```python
from build123d import *

# Parameters (mm, degrees)
V3_BOX_FOOTPRINT_100_X_45_MM_W                 = 100
V3_BOX_FOOTPRINT_100_X_45_MM_H                 = 45
V3_BOX_HEIGHT_35_MM_DEPTH                      = 35
V3_REAR_OPENING_96_X_31_MM_W                   = 96
V3_REAR_OPENING_96_X_31_MM_H                   = 31
V3_CAVITY_ALL_WALLS_2_MM_DEPTH                 = 43
V3_SQUARE_BEAMS_10_X_10_PITCH_95_MM_W          = 10
V3_SQUARE_BEAMS_10_X_10_PITCH_95_MM_H          = 10
V3_FORWARD_BEAM_LENGTH_65_MM_DEPTH             = 65
V3_LEFT_PCB_EAR_PROFILE_W                      = 10
V3_LEFT_PCB_EAR_PROFILE_H                      = 10
V3_LEFT_INWARD_EAR_5_MM_DEPTH                  = 5
V3_RIGHT_PCB_EAR_PROFILE_W                     = 10
V3_RIGHT_PCB_EAR_PROFILE_H                     = 10
V3_RIGHT_INWARD_EAR_5_MM_DEPTH                 = 5
V3_PCB_ROOF_PAIR_PITCH_85_MM_R                 = 1.7
V3_M3_ROOF_HOLES_DIAMETER_3_4_MM_DEPTH         = 2
V3_PCB_FORWARD_PAIR_ROW_SPACING_60_MM_R        = 1.7
V3_M3_PCB_EAR_HOLES_DEPTH                      = 10
V3_CHASSIS_TOP_HOLES_WIDTH_95_DEPTH_40_M_R     = 1.7
V3_M3_BEAM_TOP_BOTTOM_HOLES_DEPTH              = 10
V3_HANGING_PLATE_OFFSET_26_THICKNESS_2_5_W     = 110
V3_HANGING_PLATE_OFFSET_26_THICKNESS_2_5_H     = 2.5
V3_MOUNTING_PLATE_DOWNWARD_15_MM_WIDTH_1_DEPTH = 15
V3_FOUR_MOUNTING_SLOTS_3_4_X_10_MM_DEPTH       = 2.5


with BuildPart() as part:
    # V3 box footprint 100 x 45 mm → V3 box height 35 mm (new body)
    with BuildSketch(Plane.XY):
        with Locations((0, 22.5)):
            Rectangle(V3_BOX_FOOTPRINT_100_X_45_MM_W, V3_BOX_FOOTPRINT_100_X_45_MM_H)
    extrude(amount=V3_BOX_HEIGHT_35_MM_DEPTH)

    # V3 rear opening 96 x 31 mm → V3 cavity all walls 2 mm (cut)
    with BuildSketch(Plane(origin=(0, 45, 0), x_dir=(1, 0, 0), z_dir=(0, 1, 0))):
        with Locations((0, -17.5)):
            Rectangle(V3_REAR_OPENING_96_X_31_MM_W, V3_REAR_OPENING_96_X_31_MM_H)
    extrude(amount=-V3_CAVITY_ALL_WALLS_2_MM_DEPTH, mode=Mode.SUBTRACT)

    # V3 square beams 10 x 10 pitch 95 mm → V3 forward beam length 65 mm (add)
    with BuildSketch(Plane.XZ):
        with Locations((-47.5, 30)):
            Rectangle(V3_SQUARE_BEAMS_10_X_10_PITCH_95_MM_W, V3_SQUARE_BEAMS_10_X_10_PITCH_95_MM_H)
        with Locations((47.5, 30)):
            Rectangle(V3_SQUARE_BEAMS_10_X_10_PITCH_95_MM_W, V3_SQUARE_BEAMS_10_X_10_PITCH_95_MM_H)
    extrude(amount=V3_FORWARD_BEAM_LENGTH_65_MM_DEPTH)

    # V3 left PCB ear profile → V3 left inward ear 5 mm (add)
    with BuildSketch(Plane(origin=(-42.5, 0, 0), x_dir=(0, 0, -1), z_dir=(1, 0, 0))):
        with Locations((-30, -20)):
            Rectangle(V3_LEFT_PCB_EAR_PROFILE_W, V3_LEFT_PCB_EAR_PROFILE_H)
    extrude(amount=V3_LEFT_INWARD_EAR_5_MM_DEPTH)

    # V3 right PCB ear profile → V3 right inward ear 5 mm (add)
    with BuildSketch(Plane.ZY.offset(-42.5)):
        with Locations((30, -20)):
            Rectangle(V3_RIGHT_PCB_EAR_PROFILE_W, V3_RIGHT_PCB_EAR_PROFILE_H)
    extrude(amount=V3_RIGHT_INWARD_EAR_5_MM_DEPTH)

    # V3 PCB roof pair pitch 85 mm → V3 M3 roof holes diameter 3.4 mm (cut)
    with BuildSketch(Plane.XY.offset(35)):
        with Locations((-42.5, 40)):
            Circle(V3_PCB_ROOF_PAIR_PITCH_85_MM_R)
        with Locations((42.5, 40)):
            Circle(V3_PCB_ROOF_PAIR_PITCH_85_MM_R)
    extrude(amount=-V3_M3_ROOF_HOLES_DIAMETER_3_4_MM_DEPTH, mode=Mode.SUBTRACT)

    # V3 PCB forward pair row spacing 60 mm → V3 M3 PCB ear holes (cut)
    with BuildSketch(Plane.XY.offset(35)):
        with Locations((-42.5, -20)):
            Circle(V3_PCB_FORWARD_PAIR_ROW_SPACING_60_MM_R)
        with Locations((42.5, -20)):
            Circle(V3_PCB_FORWARD_PAIR_ROW_SPACING_60_MM_R)
    extrude(amount=-V3_M3_PCB_EAR_HOLES_DEPTH, mode=Mode.SUBTRACT)

    # V3 chassis top holes width 95 depth 40 mm → V3 M3 beam top bottom holes (cut)
    with BuildSketch(Plane.XY.offset(35)):
        with Locations((-47.5, -55)):
            Circle(V3_CHASSIS_TOP_HOLES_WIDTH_95_DEPTH_40_M_R)
        with Locations((-47.5, -15)):
            Circle(V3_CHASSIS_TOP_HOLES_WIDTH_95_DEPTH_40_M_R)
        with Locations((47.5, -55)):
            Circle(V3_CHASSIS_TOP_HOLES_WIDTH_95_DEPTH_40_M_R)
        with Locations((47.5, -15)):
            Circle(V3_CHASSIS_TOP_HOLES_WIDTH_95_DEPTH_40_M_R)
    extrude(amount=-V3_M3_BEAM_TOP_BOTTOM_HOLES_DEPTH, mode=Mode.SUBTRACT)

    # V3 hanging plate offset 26 thickness 2.5 mm → V3 mounting plate downward 15 mm width 110 (add)
    with BuildSketch(Plane(origin=(0, 0, 25), x_dir=(-1, 0, 0), z_dir=(0, 0, -1))):
        with Locations((0, -27.25)):
            Rectangle(V3_HANGING_PLATE_OFFSET_26_THICKNESS_2_5_W, V3_HANGING_PLATE_OFFSET_26_THICKNESS_2_5_H)
    extrude(amount=V3_MOUNTING_PLATE_DOWNWARD_15_MM_WIDTH_1_DEPTH)

    # V3 slots 6 mm below beam underside centers 20 and 50 → V3 four mounting slots 3.4 x 10 mm (cut)
    with BuildSketch(Plane.XZ.offset(28.5)):
        with BuildLine():
            Line((-51.7, 15.7), (-51.7, 22.3))
            ThreePointArc((-51.7, 22.3), (-50, 24), (-48.3, 22.3))
            Line((-48.3, 22.3), (-48.3, 15.7))
            ThreePointArc((-48.3, 15.7), (-50, 14), (-51.7, 15.7))
        make_face()
        with BuildLine():
            Line((-21.7, 15.7), (-21.7, 22.3))
            ThreePointArc((-21.7, 22.3), (-20, 24), (-18.3, 22.3))
            Line((-18.3, 22.3), (-18.3, 15.7))
            ThreePointArc((-18.3, 15.7), (-20, 14), (-21.7, 15.7))
        make_face()
        with BuildLine():
            Line((18.3, 15.7), (18.3, 22.3))
            ThreePointArc((18.3, 22.3), (20, 24), (21.7, 22.3))
            Line((21.7, 22.3), (21.7, 15.7))
            ThreePointArc((21.7, 15.7), (20, 14), (18.3, 15.7))
        make_face()
        with BuildLine():
            Line((48.3, 15.7), (48.3, 22.3))
            ThreePointArc((48.3, 22.3), (50, 24), (51.7, 22.3))
            Line((51.7, 22.3), (51.7, 15.7))
            ThreePointArc((51.7, 15.7), (50, 14), (48.3, 15.7))
        make_face()
    extrude(amount=-V3_FOUR_MOUNTING_SLOTS_3_4_X_10_MM_DEPTH, mode=Mode.SUBTRACT)


solid = part.part
```
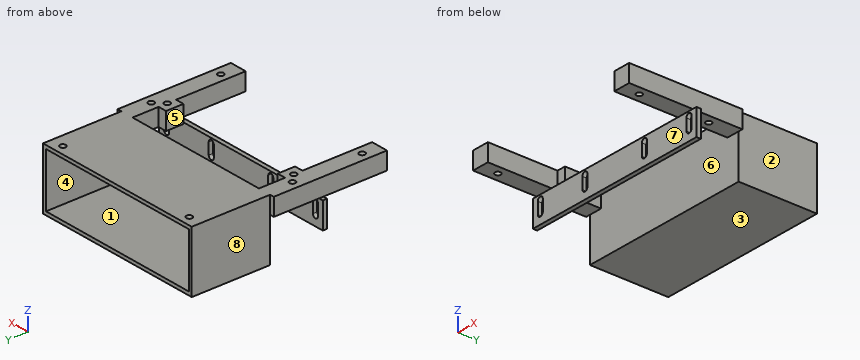
Geometry: final body of the model. Coordinates: model frame, mm. Face numbers are marked on the shaded views. A direction names the side the tool comes from. Coordinates: 2 decimals unless noted, no trailing zeros. Order: outer loops, then holes, each group sorted by start corner. A loop starts at its lowest first (then second) coordinate and runs counter-clockwise, first axis right, second up. Notation, with made-up numbers: M 43.5,52 L 67.5,52 A19 cw 67.5,74 Z; hole C 16.25,-10.75 d9. An arc over 180 degrees is marked long. Answer in a Markdown table with one row per item. Add a question column.
Q1. Section query C-C on z = 17. Return the cut outline in (x, y), and give its area (3 significant figures).
Q2. Section query A-A on y = -45. Return the cut outline in (x, z), and give its area (3 significant figures).
Q3. Contact query for flat-ended pins moving along their axis: P1, Ø0.8, axis at x = -54, y = -27, coming from the +Z side; P2, Ø4, axis at x = -40, z = 28, coming from the +Y side; P3, Ø3, axis at y = -10.5, z = 32, coming from the -X side; P4, Ø4, axis at x = 47.5, y = -15, coming from the +Z side. Output: stop coordinate, or through.
Q4. Mould query, pull axis Z, two halves, no side actions, for the marked faces 1, 2 and 3. Classes: released by +Z, released by -Z, zero draft, split by the parting line, or undercut.
Q5. Section query B-B on x = 25.5. Return the cut outline in (y, z).
Q6. Line query: L1, parallel to Y at x = -47.5, z = 32.75; L2, parallel to Z at x = -10.5, y = 31; L3, parallel to X at y = 24.5, z = 21.5. Output: solid intervals per line, ascending.
Q7. Reachability of the marked faces 4, 5, 6, 7 and 8 from +Z, -Z, +X, -X, +Y, -Y: full face, straight path, thin tool, end or side. Return the list, or none.
Q8. Section query D-D on y = 13.5. Return the cut outline in (x, z), and give its area (3 significant figures).
Completed:
| question | item | result |
|---|---|---|
| 1 | outline | M -55,-28.5 L -51.7,-28.5 L -51.7,-26 L -55,-26 Z; M -50,0 L 50,0 L 50,45 L 48,45 L 48,2 L -48,2 L -48,45 L -50,45 Z; M -48.3,-28.5 L -21.7,-28.5 L -21.7,-26 L -48.3,-26 Z; M -18.3,-28.5 L 18.3,-28.5 L 18.3,-26 L -18.3,-26 Z; M 21.7,-28.5 L 48.3,-28.5 L 48.3,-26 L 21.7,-26 Z; M 51.7,-28.5 L 55,-28.5 L 55,-26 L 51.7,-26 Z |
| 1 | area | 613 mm2 |
| 2 | outline | M -52.5,25 L -42.5,25 L -42.5,35 L -52.5,35 Z; M 42.5,25 L 52.5,25 L 52.5,35 L 42.5,35 Z |
| 2 | area | 200 mm2 |
| 3 | P1 | stops at z = 25 |
| 3 | P2 | stops at y = 2 |
| 3 | P3 | stops at x = -52.5 |
| 3 | P4 | stops at z = 35 |
| 4 | face 1 | undercut |
| 4 | face 2 | zero draft |
| 4 | face 3 | released by -Z |
| 5 | outline | M -28.5,10 L -26,10 L -26,25 L -28.5,25 Z; M 0,0 L 45,0 L 45,2 L 2,2 L 2,33 L 45,33 L 45,35 L 0,35 Z |
| 6 | L1 | y = -65 to -56.7, -53.3 to -16.7, -13.3 to 2 |
| 6 | L2 | z = 0 to 2, 33 to 35 |
| 6 | L3 | x = -50 to -48, 48 to 50 |
| 7 | face 4 | +Y |
| 7 | face 5 | +Z, -Z, -Y |
| 7 | face 6 | -Z |
| 7 | face 7 | -Z, +X, -X, -Y |
| 7 | face 8 | +Z, -Z, -X, +Y |
| 8 | outline | M -50,0 L 50,0 L 50,35 L -50,35 Z; hole M -48,2 L 48,2 L 48,33 L -48,33 Z |
| 8 | area | 524 mm2 |
